Design review of the part built by this model. Coordinates are the model's own, in mm. Face numbers are marked on the shaded views. A direction names the side the tool comes from. Coordinates: 2 decimals unless noted, no trailing zeros. Loops run counter-clockwise (first coordinate to the right, second up) from the corner with the lowest first, then second, coordinate; pieces in that order, holes last. Notation, with made-up numbers: (-24.5, 52) -> (21.5, 52) arc R26 ccw to (21.5, 81) -> close; hole circle Ø8 at (57.25, -10). An arc over 180 degrees is marked (long way). One line per item, written item: value. Start each with the question number.
1. Add section C-C on x = -14. Write out the cut boundary in (y, z).
2. Insertion check: pin 1 (10 mm diameter, centred on x = 2.5, z = 4, fed in from +Y); pin 2 (15.5 mm diameter, centred on x = 3.5, z = -3.5, fed in from -Y); pin 3 (7.5 mm diameter, centred on x = 0, z = 0, fed in from -Y). Each pin has a flat end and moves straight along its axis. Give the tip position at first contact, or say it passes through.
3. Add section A-A on z = 14.5. Write out the cut boundary in (x, y).
4. Add section D-D on x = 13.65. Write out the cut boundary in (y, z).
5. Machinability: for the marked faces 1, 2 and 3, which of the approach directions +Z, -Z, +X, -X, +Y, -Y give a long, thin tool a straight path to every point of the face, cutting with its end or side? Answer none if there is none.
6. For probe 1 along X at (y, z) = (-3.3, 0); probe 2 along X at (y, z) = (-3.75, 5.5); probe 3 along Z at (x, y) = (0, -2.6), list the stretches that pass through material, from the lowest coordinate up.
7. Add section B-B on y = -4. Write out the cut boundary in (x, z).
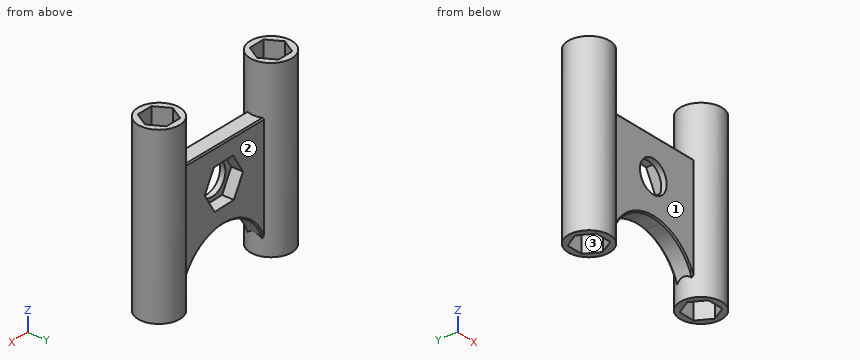
```python
from build123d import *

# Parameters (mm, degrees)
F0_R          = 3.25
F1_DEPTH      = 3.5
F3_DEPTH      = 2.4
F4_R          = 4.25
F5_DEPTH      = 17.5
F5_DEPTH_BACK = 17.5
F6_SIZE       = 0.25


with BuildPart() as f1:
    # F0 (on Front) → F1 (new body)
    with BuildSketch(Plane.XZ):
        with BuildLine():
            Line((10.3391141687, -17.4996029254), (10.25, -7.5))
            Line((10.25, -7.5), (2.081973366, -7.5))
            ThreePointArc((2.081973366, -7.5), (7.9829074445, -11.0362777063), (10.3391141687, -17.4996029254))
        make_face()
        with BuildLine():
            Line((2.081973366, -7.5), (10.25, -7.5))
            Line((10.25, -7.5), (10.25, 7.5))
            Line((10.25, 7.5), (-10.25, 7.5))
            Line((-10.25, 7.5), (-10.25, -7.5))
            Line((-10.25, -7.5), (-1.9928591974, -7.5))
            ThreePointArc((-1.9928591974, -7.5), (0.0445570843, -7.2963797866), (2.081973366, -7.5))
        make_face()
        Circle(F0_R, mode=Mode.SUBTRACT)
        with BuildLine():
            ThreePointArc((-10.25, -17.4996029254), (-7.8937932759, -11.0362777063), (-1.9928591974, -7.5))
            Line((-1.9928591974, -7.5), (-10.25, -7.5))
            Line((-10.25, -7.5), (-10.25, -17.4996029254))
        make_face()
    extrude(amount=F1_DEPTH)

    # F2 (on Front) → F3 (cut)
    with BuildSketch(Plane.XZ):
        Polygon((-2.4370454627, -3.9929711461), (2.2394917178, -4.1070288539), (4.6765371804, -0.1140577078), (2.4370454627, 3.9929711461), (-2.2394917178, 4.1070288539), (-4.6765371804, 0.1140577078), align=None)
    extrude(amount=F3_DEPTH, mode=Mode.SUBTRACT)

    # F4 (on Top) → F5 (join, two sides)
    with BuildSketch(Plane.XY) as f5_sk:
        with Locations((13.65, -1.804011694)):
            Circle(F4_R)
        Polygon((17.0274990748, -1.804011694), (15.3387495374, -4.729011694), (11.9612504626, -4.729011694), (10.2725009252, -1.804011694), (11.9612504626, 1.120988306), (15.3387495374, 1.120988306), align=None, mode=Mode.SUBTRACT)
        with Locations((-13.65, -1.804011694)):
            Circle(F4_R)
        Polygon((-11.9612504626, -4.729011694), (-15.3387495374, -4.729011694), (-17.0274990748, -1.804011694), (-15.3387495374, 1.120988306), (-11.9612504626, 1.120988306), (-10.2725009252, -1.804011694), align=None, mode=Mode.SUBTRACT)
    extrude(amount=F5_DEPTH)
    extrude(f5_sk.sketch, amount=-F5_DEPTH_BACK)

    # F6
    f6_edges = [f1.edges().sort_by_distance(p)[0] for p in [
        (0, -3.5, 7.5),
        (0, 0, 7.5),
        (-0.094724, -3.5, -7.297322),
        (-0.101304, 0, -7.297413),
    ]]
    chamfer(f6_edges, length=F6_SIZE)


solid = f1.part
```
Worked answers:
1. outline: (-6.04, -17.5) -> (-4.73, -17.5) -> (-4.73, 17.5) -> (-6.04, 17.5) -> close; (1.12, -17.5) -> (2.43, -17.5) -> (2.43, 17.5) -> (1.12, 17.5) -> close
2. pin 1: stops at y = 0
2. pin 2: stops at y = -5.31
2. pin 3: stops at y = -3.5
3. outline: circle Ø8.5 at (-13.65, -1.8); circle Ø8.5 at (13.65, -1.8); hole (-17.03, -1.8) -> (-15.34, -4.73) -> (-11.96, -4.73) -> (-10.27, -1.8) -> (-11.96, 1.12) -> (-15.34, 1.12) -> close; hole (10.27, -1.8) -> (11.96, -4.73) -> (15.34, -4.73) -> (17.03, -1.8) -> (15.34, 1.12) -> (11.96, 1.12) -> close
4. outline: (-6.05, -17.5) -> (-4.73, -17.5) -> (-4.73, 17.5) -> (-6.05, 17.5) -> close; (1.12, -17.5) -> (2.45, -17.5) -> (2.45, 17.5) -> (1.12, 17.5) -> close
5. face 1: +Z, -Z, -Y
5. face 2: +Z, -Z, +Y
5. face 3: +Z, -Z
6. probe 1: x = -17.63 to -16.16, -11.14 to -3.25, 3.25 to 11.14, 16.16 to 17.63
6. probe 2: x = -17.43 to -15.9, -11.4 to -9.87, 9.87 to 11.4, 15.9 to 17.43
6. probe 3: z = -7.3 to -3.25, 3.25 to 7.5
7. outline: (-17.29, -17.5) -> (-15.76, -17.5) -> (-15.76, 17.5) -> (-17.29, 17.5) -> close; (-11.54, -17.5) -> (-10.01, -17.5) -> (-10.01, 17.5) -> (-11.54, 17.5) -> close; (10.01, -17.5) -> (11.54, -17.5) -> (11.54, 17.5) -> (10.01, 17.5) -> close; (15.76, -17.5) -> (17.29, -17.5) -> (17.29, 17.5) -> (15.76, 17.5) -> close
